Here's how the part is built. I have some questions about the finished solid (model axes, mm). A direction names the side the tool comes from. Round coordinates to 2 decimals unless told otherwise and drop trailing zeros. Order: outer loops, then holes, each group sorted by start corner. A loop starts at its lowest first (then second) coordinate and runs counter-clockwise, first axis right, second up. Notation, with made-up numbers: (26, 85) -> (47, 85) arc R10 cw to (47, 90) -> close; hole circle Ø3 at (56, -31.5). An arc over 180 degrees is marked (long way). Answer in a Markdown table with one row per item.
Autodesk Inventor part; units mm, degrees
ref_plane "YZ Plane" through (0, 0, 0) normal (1, 0, 0) x (0, 1, 0)
ref_plane "XZ Plane" through (0, 0, 0) normal (0, 1, 0) x (-1, 0, 0)
ref_plane "XY Plane" through (0, 0, 0) normal (0, 0, 1) x (1, 0, 0)
sketch "Skizze1" plane through (0, 0, 0) normal (0, 1, 0) x (-1, 0, 0)
  line L0 (5, 20) -> (-15, 20)
  line L1 (-15, 20) -> (-15, -20)
  line L2 (-15, -20) -> (5, -20)
  line L3 (5, -20) -> (5, 20)
  line L4 (0, 15) -> (0, -15) construction
  line L5 (5, 0) -> (0, 0) construction
  circle A0 centre (0, -15) radius 3
  circle A1 centre (0, 15) radius 3
  dimension "d0" = 30
  dimension "d1" = 40
  dimension "d2" = 6
  dimension "d5" = 5
  dimension "d6" = 15
extrude "Extrusion1" add sketch "Skizze1" along normal mid plane 10
sketch "Skizze2" plane through (15, -5, -20) normal (1, 0, 0) x (0, 0, -1)
  circle A0 centre (-20, 5) radius 3
  dimension "d7" = 6
extrude "Extrusion2" cut sketch "Skizze2" against normal through all
sketch "Skizze3" plane through (-5, 5, 20) normal (0, 0, 1) x (1, 0, 0)
  line L0 (20, -10) -> (20, 0)
  line L1 (20, -5) -> (15, -5) construction
  point P0 (5, -5)
  dimension "d10" = 5
hole "Bohrung1" at (10, 0, 20) direction (0, 0, -1) diameter 3.242 depth 14 tip angle 118
sketch "Skizze4" plane through (-5, 5, 20) normal (0, 0, 1) x (1, 0, 0)
  point P0 (5, -5)
hole "Bohrung2" at (0, 0, 20) direction (0, 0, -1) diameter 1.567 depth 6.3 tip angle 118
mirror "Spiegeln2" about plane through (0, 0, 0) normal (0, 0, 1) of "Bohrung2"
sketch "Skizze5" plane through (15, -5, -20) normal (1, 0, 0) x (0, 0, -1)
  circle A0 centre (-20, 5) radius 3
  line L0 (0, 0) -> (0, 10)
  line L1 (-40, 10) -> (0, 10)
  line L2 (-40, 0) -> (-40, 10)
  line L3 (0, 0) -> (-40, 0)
  line L4 (-40, 0) -> (-40, 10)
  line L5 (-40, 10) -> (0, 10)
  line L6 (-40, 0) -> (-25, 0)
  line L7 (-25, 0) -> (-25, 10)
  line L8 (-25, 10) -> (-40, 10)
  line L9 (-40, 10) -> (-40, 0)
  dimension "d25" = 15
extrude "Extrusion3" add sketch "Skizze5" along normal blind 12 contours L3 L2 L1 L7
sketch "Skizze6" plane through (0, 5, 0) normal (0, 1, 0) x (1, 0, 0)
  circle A0 centre (0, -15) radius 3
  circle A1 centre (0, 15) radius 3
  line L0 (-5, -20) -> (27, -20)
  line L1 (27, -5) -> (27, -20)
  line L2 (15, -5) -> (27, -5)
  line L3 (15, -5) -> (15, 20)
  line L4 (15, 20) -> (-5, 20)
  line L5 (-5, 20) -> (-5, -20)
  line L6 (15, -5) -> (15, 20) construction
  circle A2 centre (19.5, -12.5) radius 5.05
  line L7 (27, -5) -> (27, -20)
  line L8 (27, -12.5) -> (19.5, -12.5) construction
  line L9 (25.2991, -5) -> (25.2991, -12.5) construction
  point P0 (0, 0)
  dimension "d28" = 10.1
extrude "Extrusion4" cut sketch "Skizze6" against normal blind 6 contours A2
sketch "Skizze7" plane through (0, 5, 0) normal (0, 1, 0) x (1, 0, 0)
  circle A0 centre (19.5, -12.5) radius 5.05
  circle A1 centre (0, -15) radius 3
  circle A2 centre (0, 15) radius 3
  line L0 (-5, -20) -> (27, -20)
  line L1 (27, -5) -> (27, -20)
  line L2 (15, -5) -> (27, -5)
  line L3 (15, -5) -> (15, 20)
  line L4 (15, 20) -> (-5, 20)
  line L5 (-5, 20) -> (-5, -20)
  line L6 (27, -5) -> (27, -20)
  line L7 (27, -14.5) -> (17.9872, -14.5)
  line L8 (17.9872, -14.5) -> (17.9872, -10.5)
  line L9 (17.9872, -10.5) -> (27, -10.5)
  line L10 (27, -10.5) -> (27, -14.5)
  point P0 (0, 0)
  point P1 (27, -12.5)
  dimension "d37" = 4
sketch "Skizze8" plane through (15, -5, -20) normal (1, 0, 0) x (0, 0, -1)
  line L0 (-25, 10) -> (-25, 0)
  line L1 (0, 0) -> (-25, 0)
  line L2 (0, 0) -> (0, 10)
  line L3 (-25, 10) -> (0, 10)
  circle A0 centre (-20, 5) radius 3
  line L4 (0, 0) -> (-10, 0)
  line L5 (-10, 0) -> (-10, 10)
  line L6 (-10, 10) -> (0, 10)
  line L7 (0, 10) -> (0, 0)
  dimension "d31" = 10
extrude "Extrusion5" add sketch "Skizze8" along normal blind 10 contours L3 L2 L1 L5
sketch "Skizze9" plane through (25, -5, -20) normal (1, 0, 0) x (0, 0, -1)
  line L0 (0, 0) -> (0, 10)
  line L1 (0, 10) -> (-10, 10)
  line L2 (-10, 10) -> (-10, 0)
  line L3 (-10, 0) -> (0, 0)
  line L4 (-10, 2) -> (0, 2)
  line L5 (0, 2) -> (0, 8)
  line L6 (0, 8) -> (-10, 8)
  line L7 (-10, 8) -> (-10, 2)
  point P0 (-20, 5)
  point P1 (0, 5)
  dimension "d34" = 6
extrude "Extrusion6" cut sketch "Skizze9" against normal blind 6 contours L4 L2 L6 L0
extrude "Extrusion7" cut sketch "Skizze7" against normal up to surface (6 mm away) contours A0 L7 L8 L9 | A0 L9 L1 L7 picked at (20.1748, -12.5)
properties part number "Probenkammer Halter Plus-Seite" material "Aluminium 6061"
1. Suppose I cut it at D-D on x = 13.5. Write out the boundary of the cut face in (y, z).
Numbers:
| item | result |
|---|---|
| outline | (-5, -20) -> (5, -20) -> (5, 20) -> (-5, 20) -> close; hole circle Ø6 at (0, 0) |
2. Suppose I cut it at C-C on z = 0. Write out the boundary of the cut face in (x, y).
Numbers:
| item | result |
|---|---|
| outline | (-5, -5) -> (15, -5) -> (15, -3) -> (-5, -3) -> close; (-5, 3) -> (15, 3) -> (15, 5) -> (-5, 5) -> close |
3. For pin 1 Ø5 at (y, z) = (0.5, -3.5) entering from +X; pin 2 Ø3.5 at (x, z) = (0, -15) entering from -Y; pin 3 Ø0.6 at (y, z) = (-3.5, -16) entering from +X; pin 4 Ø3 at (y, z) = (1, -16) entering from +X, each with a flat end and sliding along its axis, tell me the tip position at first contact or that it passes through.
Numbers:
| item | result |
|---|---|
| pin 1 | stops at x = 15 |
| pin 2 | passes through |
| pin 3 | stops at x = 25 |
| pin 4 | stops at x = 19 |
4. Suppose I cut it at B-B on x = 0. Write out the boundary of the cut face in (y, z).
Numbers:
| item | result |
|---|---|
| outline | (-5, -20) -> (-0.78, -20) -> (-0.78, -18) -> (-5, -18) -> close; (-5, -12) -> (5, -12) -> (5, 12) -> (-5, 12) -> close; (-5, 18) -> (-0.78, 18) -> (-0.78, 20) -> (-5, 20) -> close; (0.78, -20) -> (5, -20) -> (5, -18) -> (0.78, -18) -> close; (0.78, 18) -> (5, 18) -> (5, 20) -> (0.78, 20) -> close; hole circle Ø6 at (0, 0) |
5. We'd pull the mould along X, two halves only. Please class faces 4 (the face through (18.8, -0.1, -10)), 5 (the face through (10.279, 0.037, 5.195)), 6 (the face through (27, -2, 13)): released by +X, released by -X, zero draft, split by the parting line, or undercut.
Numbers:
| item | result |
|---|---|
| face 4 | zero draft |
| face 5 | undercut |
| face 6 | released by +X |
6. Please list where these lines run through material, in increasing order: line 1 along Z through (x, y) = (19.5, 3.35); line 2 along Z through (x, y) = (18, -4); line 3 along Y through (x, z) = (19.5, -12.5).
Numbers:
| item | result |
|---|---|
| line 1 | z = -20 to -10, 5 to 7.45, 17.55 to 20 |
| line 2 | z = -20 to -10, 5 to 20 |
| line 3 | y = -5 to -3, 3 to 5 |
7. Suppose I cut it at A-A on z = -15. Write out the boundary of the cut face in (x, y).
Numbers:
| item | result |
|---|---|
| outline | (-5, -5) -> (-3, -5) -> (-3, 5) -> (-5, 5) -> close; (3, -5) -> (25, -5) -> (25, -3) -> (19, -3) -> (19, 3) -> (25, 3) -> (25, 5) -> (3, 5) -> close |
8. For faces 1 (the face through (0.235, -0.747, -18.933)), 2 (the face through (15, 0, -4)), 3 (the face through (26, 2, 14.5)), which set-ups out of +Z, -Z, +X, -X, +Y, -Y let a thin tool reach every point of the face, with its end or its side?
Numbers:
| item | result |
|---|---|
| face 1 | -Z |
| face 2 | +X, +Y, -Y |
| face 3 | +X, +Y |
